For this review, take the finished solid that the model builds, in its own axes (mm). Face numbers are marked on the shaded views. A direction names the side the tool comes from. Give positions to 0.01 mm unless a question says otherwise; leave off trailing zeros. Loops run counter-clockwise (first coordinate to the right, second up) from the corner with the lowest first, then second, coordinate; pieces in that order, holes last.
```python
from build123d import *

# Parameters (mm, degrees)
SKETCH1_W           = 89
SKETCH1_H           = 192
BOSS_EXTRUDE1_DEPTH = 30
SKETCH2_R           = 34.99943994
CUT_EXTRUDE1_DEPTH  = 10
SKETCH3_W           = 75
SKETCH3_H           = 5
CUT_EXTRUDE2_DEPTH  = 102
CUT_EXTRUDE4_DEPTH  = 102
SKETCH6_W           = 10.5
SKETCH6_H           = 4
CUT_EXTRUDE7_DEPTH  = 8
BOSS_EXTRUDE2_DEPTH = 10.5
CUT_EXTRUDE8_DEPTH  = 20.767757578
BOSS_EXTRUDE3_DEPTH = 10.5
CUT_EXTRUDE9_DEPTH  = 22.812544275
BOSS_EXTRUDE6_DEPTH = 10.5
BOSS_EXTRUDE7_DEPTH = 10.5
FILLET1_R           = 10
FILLET2_R           = 10
FILLET3_R           = 10
FILLET4_R           = 10
CUT_EXTRUDE11_DEPTH = 99
SKETCH15_W          = 7.554212703
SKETCH15_H          = 3.259234926
CUT_EXTRUDE12_DEPTH = 99
FILLET5_R           = 10
SKETCH16_W          = 51.485854904
SKETCH16_H          = 41.780762453
CUT_EXTRUDE13_DEPTH = 221


with BuildPart() as part:
    # Sketch1 → Boss-Extrude1 (new body)
    with BuildSketch(Plane(origin=(0, 0, 0), x_dir=(1, 0, 0), z_dir=(0, 1, 0))):
        with Locations((-10.5, 20.043668932)):
            Rectangle(SKETCH1_W, SKETCH1_H)
        with BuildLine():
            Line((-44.5, -34.956331068), (-44.5, 75.043668932))
            ThreePointArc((-44.5, 75.043668932), (-10.5, 109.043668932), (23.5, 75.043668932))
            Line((23.5, 75.043668932), (23.5, -34.956331068))
            ThreePointArc((23.5, -34.956331068), (-10.5, -68.956331068), (-44.5, -34.956331068))
        make_face(mode=Mode.SUBTRACT)
    extrude(amount=BOSS_EXTRUDE1_DEPTH)

    # Sketch2 → Cut-Extrude1 (cut)
    with BuildSketch(Plane.XZ):
        with Locations((-10.5, 37.838844027)):
            Circle(SKETCH2_R)
    extrude(amount=-CUT_EXTRUDE1_DEPTH, mode=Mode.SUBTRACT)

    # Sketch3 → Cut-Extrude2 (cut)
    with BuildSketch(Plane(origin=(34, 0, 0), x_dir=(0, 0, -1), z_dir=(1, 0, 0))):
        with Locations((-34.286288065, 12.5)):
            Rectangle(SKETCH3_W, SKETCH3_H)
    extrude(amount=-CUT_EXTRUDE2_DEPTH, mode=Mode.SUBTRACT)

    # Sketch4 → Cut-Extrude4 (cut)
    with BuildSketch(Plane.ZY.offset(55)):
        Polygon((-40.970715348, 29.469395922), (-41.211628541, 24.561719678), (-3.213711935, 10), (-3.213711935, 15), align=None)
    extrude(amount=-CUT_EXTRUDE4_DEPTH, mode=Mode.SUBTRACT)

    # Sketch6 → Cut-Extrude7 (cut)
    with BuildSketch(Plane(origin=(0, 30, 0), x_dir=(1, 0, 0), z_dir=(0, 1, 0))):
        with Locations((-49.75, 40.570603007)):
            Rectangle(SKETCH6_W, SKETCH6_H)
        with Locations((28.75, 40.570603007)):
            Rectangle(SKETCH6_W, SKETCH6_H)
    extrude(amount=-CUT_EXTRUDE7_DEPTH, mode=Mode.SUBTRACT)

    # Sketch7 → Boss-Extrude2 (add)
    with BuildSketch(Plane.ZY.offset(55)):
        Polygon((-38.570603007, 23.549614886), (-42.570603007, 25.082511526), (-42.570603007, 22), (-38.570603007, 22), align=None)
    extrude(amount=-BOSS_EXTRUDE2_DEPTH)

    # Sketch8 → Cut-Extrude8 (cut)
    with BuildSketch(Plane.ZY.offset(55)):
        Polygon((-42.570603007, 25.082511526), (-55.402488324, 30), (-42.570603007, 30), align=None)
    extrude(amount=-CUT_EXTRUDE8_DEPTH, mode=Mode.SUBTRACT)

    # Sketch9 → Boss-Extrude3 (add)
    with BuildSketch(Plane(origin=(34, 0, 0), x_dir=(0, 0, -1), z_dir=(1, 0, 0))):
        Polygon((38.570603007, 23.549614886), (42.570603007, 25.082511526), (42.570603007, 22), (38.570603007, 22), align=None)
    extrude(amount=-BOSS_EXTRUDE3_DEPTH)

    # Sketch10 → Cut-Extrude9 (cut)
    with BuildSketch(Plane(origin=(34, 0, 0), x_dir=(0, 0, -1), z_dir=(1, 0, 0))):
        Polygon((42.570603007, 25.082511526), (55.402488324, 30), (42.570603007, 30), align=None)
    extrude(amount=-CUT_EXTRUDE9_DEPTH, mode=Mode.SUBTRACT)

    # Sketch12 → Boss-Extrude6 (add)
    with BuildSketch(Plane.ZY.offset(55)):
        Polygon((-38.570603007, 30), (-41.570603007, 30), (-38.570603007, 28.549614886), align=None)
    extrude(amount=-BOSS_EXTRUDE6_DEPTH)

    # Sketch11 → Boss-Extrude7 (add)
    with BuildSketch(Plane(origin=(34, 0, 0), x_dir=(0, 0, -1), z_dir=(1, 0, 0))):
        Polygon((38.570603007, 28.549614886), (41.570603007, 30.007074027), (38.570603007, 30), align=None)
    extrude(amount=-BOSS_EXTRUDE7_DEPTH)

    # Fillet1
    fillet1_edges = [part.edges().sort_by_distance(p)[0] for p in [
        (-49.75, 30, -55.402488324),
    ]]
    fillet(fillet1_edges, radius=FILLET1_R)

    # Fillet2
    fillet2_edges = [part.edges().sort_by_distance(p)[0] for p in [
        (28.75, 30, -55.402488324),
    ]]
    fillet(fillet2_edges, radius=FILLET2_R)

    # Fillet3
    fillet3_edges = [part.edges().sort_by_distance(p)[0] for p in [
        (-49.75, 10, -3.213711935),
    ]]
    fillet(fillet3_edges, radius=FILLET3_R)

    # Fillet4
    fillet4_edges = [part.edges().sort_by_distance(p)[0] for p in [
        (28.75, 10, -3.213711935),
    ]]
    fillet(fillet4_edges, radius=FILLET4_R)

    # Sketch14 → Cut-Extrude11 (cut)
    with BuildSketch(Plane(origin=(34, 0, 0), x_dir=(0, 0, -1), z_dir=(1, 0, 0))):
        Polygon((42.717415751, 25.138773717), (116.043668932, 25.138773717), (116.043668932, 30), (57.252994033, 30), (53.674522762, 29.337801849), align=None)
    extrude(amount=-CUT_EXTRUDE11_DEPTH, mode=Mode.SUBTRACT)


with BuildPart() as cut_extrude11_piece_1:
    # of the separate pieces the step leaves, piece 1, a body of its own (cut_extrude11_pieces)
    add(part.part.solids().sort_by_distance((23.5, 25.138773717, -42.717415751))[0])

    # Fillet5
    fillet5_edges = [cut_extrude11_piece_1.edges().sort_by_distance(p)[0] for p in [
        (-49.75, 25.138773717, -42.717415751),
        (28.75, 25.138773717, -42.717415751),
    ]]
    fillet(fillet5_edges, radius=FILLET5_R)

    # Sketch16 → Cut-Extrude13 (cut)
    with BuildSketch(Plane(origin=(0, 0, -116.043668932), x_dir=(-1, 0, 0), z_dir=(0, 0, -1))):
        with Locations((36.242927452, 18.346859621)):
            Rectangle(SKETCH16_W, SKETCH16_H)
    extrude(amount=-CUT_EXTRUDE13_DEPTH, mode=Mode.SUBTRACT)


with BuildPart() as cut_extrude11_piece_2:
    # of the separate pieces the step leaves, piece 2, a body of its own (cut_extrude11_pieces)
    add(part.part.solids().sort_by_distance((23.5, 30, -57.252994033))[0])


with BuildPart() as cut_extrude11_piece_3:
    # of the separate pieces the step leaves, piece 3, a body of its own (cut_extrude11_pieces)
    add(part.part.solids().sort_by_distance((-55, 30, -57.252994033))[0])


with BuildPart() as cut_extrude12_tool:
    # Sketch15 → Cut-Extrude12 (new body)
    with BuildSketch(Plane(origin=(34, 0, 0), x_dir=(0, 0, -1), z_dir=(1, 0, 0))):
        with Locations((54.846987071, 29.864387296)):
            Rectangle(SKETCH15_W, SKETCH15_H)
    extrude(amount=-CUT_EXTRUDE12_DEPTH)


with BuildPart() as cut_extrude11_piece_2_1:
    add(cut_extrude11_piece_2.part)

    # Cut-Extrude12: cut by cut_extrude12_tool
    add(cut_extrude12_tool.part, mode=Mode.SUBTRACT)


with BuildPart() as cut_extrude11_piece_3_1:
    add(cut_extrude11_piece_3.part)

    # Cut-Extrude12: cut by cut_extrude12_tool
    add(cut_extrude12_tool.part, mode=Mode.SUBTRACT)


solid = cut_extrude11_piece_1.part
```
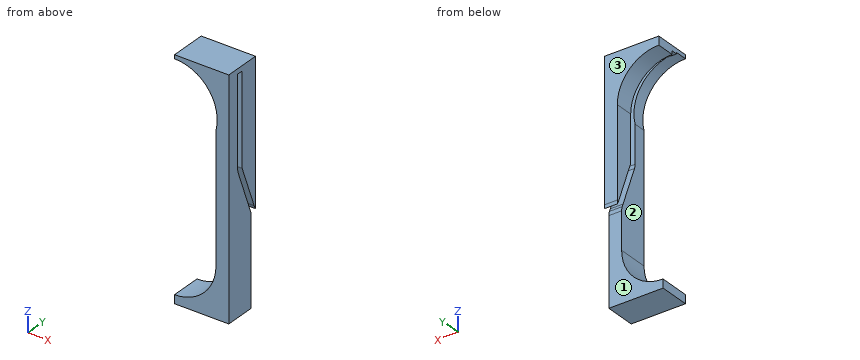
Item 1: Take a section at A-A on z = 64. Give the boundary of the cut face in (x, y).
Answer:
outline: (7.18, 15) - (34, 15) - (34, 30) - (7.18, 30) - close; (12.75, 0) - (34, 0) - (34, 10) - (12.75, 10) - close
Item 2: For L1, parallel to X at y = 8, z = -53.5; L2, parallel to Y at x = 7.5, z = -104; L3, parallel to Y at x = 25.5, z = -32, list the stretches that pass through material, from the lowest coordinate up.
Answer:
L1: x = 23.5 to 34
L2: y = 0 to 25.14
L3: y = 0 to 21.03, 26.03 to 30
Item 3: Clearance check with flat-ended pins moving along their axes: pin 1 Ø3 at (x, z) = (24, 23.5) entering from +Y; pin 2 Ø4.5 at (y, z) = (21, -17) entering from -X; pin 3 Ø6 at (y, z) = (24, -90.5) entering from -X; pin 4 Ø22.5 at (x, z) = (10.5, -5) entering from +Y. State where each tip first meets the part, or that it passes through.
Answer:
pin 1: stops at y = 30
pin 2: stops at x = 23.5
pin 3: stops at x = 18.05
pin 4: passes through
Item 4: Take a section at D-D on y = 20. Give the boundary of the cut face in (x, z).
Answer:
outline: (-10.5, -116.04) - (34, -116.04) - (34, -29.31) - (23.5, -29.31) - (23.5, -75.04) arc R34 cw to (-10.5, -109.04) - close; (-10.5, 68.96) arc R34 cw to (23.5, 34.96) - (23.5, -16.26) - (34, -16.26) - (34, 75.96) - (-10.5, 75.96) - close
Item 5: Take a section at C-C on x = -6.5. Give the boundary of the cut face in (y, z).
Answer:
outline: (0, -116.04) - (25.14, -116.04) - (25.14, -108.81) - (0, -108.81) - close; (0, 72.61) - (10, 72.61) - (10, 71.79) - (15, 71.79) - (15, 68.72) - (30, 68.72) - (30, 75.96) - (0, 75.96) - close
Item 6: Take a section at B-B on y = 6. Give the boundary of the cut face in (x, z).
Answer:
outline: (-10.5, -116.04) - (34, -116.04) - (34, 75.96) - (-10.5, 75.96) - (-10.5, 72.84) arc R35 cw to (23.5, 29.53) - (23.5, -75.04) arc R34 cw to (-10.5, -109.04) - close
Item 7: Tool access review of the marked faces 1, 2 and 3: name each direction out of +Z, -Z, +X, -X, +Y, -Y from which nothing blocks a thin tool from reaching the whole face with its end or side.
Answer:
face 1: -Z, +X, -X, +Y
face 2: -X, +Y, -Y
face 3: +Z, -Z, +X, -X, +Y
